Verification items for this drawing (mm, ordinates from the low corner). A direction names the side the tool comes from. Give positions to 0.01 mm unless a question says otherwise; leave off trailing zeros. Use a Markdown table: item, result.
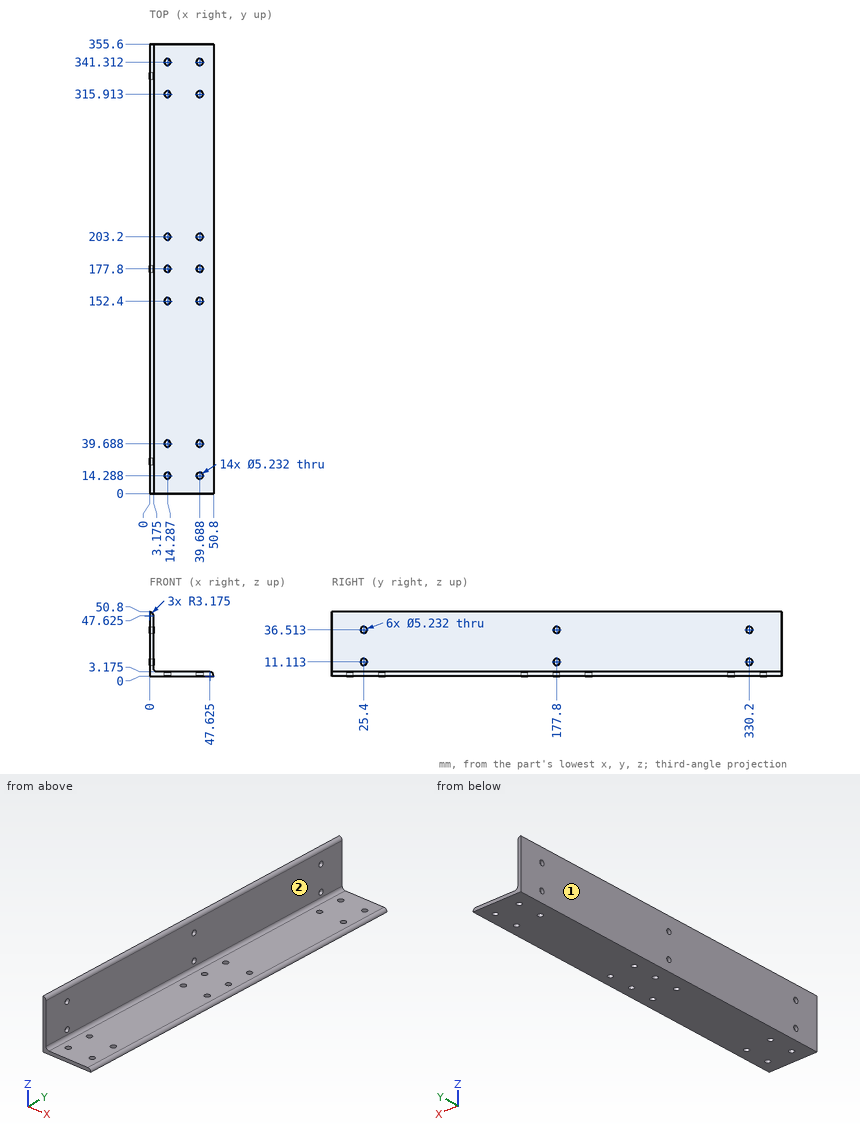
(1) Set-up check for the marked faces 1 and 2: record each of +Z, -Z, +X, -X, +Y, -Y from which the full face is reachable in a straight line by a thin tool's end or side.
Results below:
| item | result |
|---|---|
| face 1 | +Z, -Z, -X, +Y, -Y |
| face 2 | +Z, +X, +Y, -Y |
(2) Gauge pin test, flat ends, axial feed: P1, Ø6, axis at x = 14.29, y = 152.4, coming from the +Z side (1 decimal); P2, Ø6, axis at y = 330.2, z = 11.11, coming from the +X side (1 decimal). Record the tip position at first contact, or that the pin passes through.
Results below:
| item | result |
|---|---|
| P1 | z = 3.2 |
| P2 | x = 3.2 |
(3) Material ranges on line 1 (Z direction, x = 33, y = 62) (1 decimal); line 2 (Z direction, x = 1, y = 25); line 3 (Z direction, x = 1.25, y = 177.8) (1 decimal), recorded low to high.
Results below:
| item | result |
|---|---|
| line 1 | 0 to 3.2 |
| line 2 | 0 to 8.53, 13.7 to 33.93, 39.1 to 50.64 |
| line 3 | 0 to 8.5, 13.7 to 33.9, 39.1 to 50.5 |
